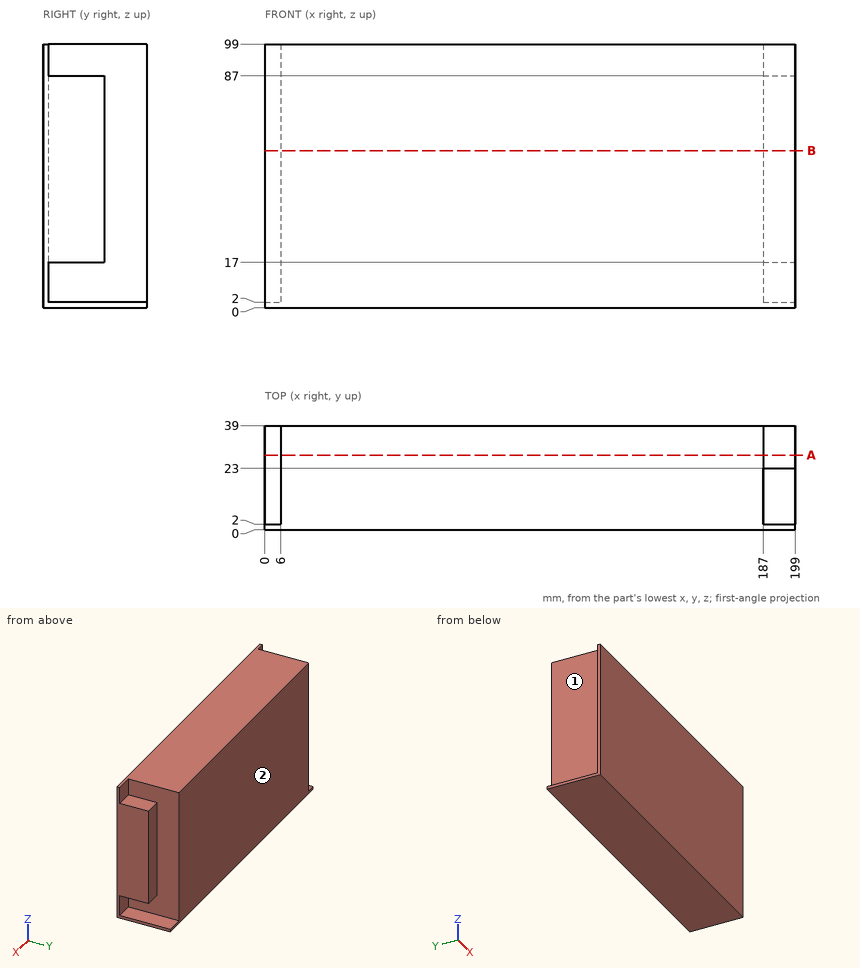
Study the drawing (mm; zero at the part's minimum x, y, z) and answer. A direction names the side the tool comes from. Round coordinates to 2 decimals unless told otherwise and drop trailing zeros. Write each loop counter-clockwise with the first axis right and the second up, starting at its lowest first coordinate (ties: lowest second). Pieces come first, ordered by that corner, then holes.
1) A cutting plane is placed at A-A on y = 28. Determine the outline of the cut face in (x, z).
2) Flat-ended cylindrical pins translate along their axes: P1, Ø13, axis at x = 195, y = 17, coming from the -Z side; P2, Ø3, axis at y = 11.5, z = 51, coming from the -X side; P3, Ø9.5, axis at x = 195.5, z = 96, coming from the +Y side; P4, Ø3.5, axis at x = 190.5, y = 14, coming from the +Z side. Find the tip coordinate at first contact, or state that the pin passes through.
3) Consider probe 1 along X at (y, z) = (17, 17.5); probe 2 along X at (y, z) = (7.5, 8.5). Determine where each line is inside the solid, lowest interval first.
4) A cutting plane is placed at B-B on z = 59. Determine the outline of the cut face in (x, y).
5) Which of the six approach directions +Z, -Z, +X, -X, +Y, -Y give full straight-line access (tool end or side, diameter ignored) to the marked faces 1 and 2?
Entries:
1. outline: (0, 0) - (199, 0) - (199, 2) - (187, 2) - (187, 99) - (6, 99) - (6, 2) - (0, 2) - close
2. P1: stops at z = 0
2. P2: stops at x = 6
2. P3: stops at y = 2
2. P4: stops at z = 87
3. probe 1: x = 6 to 199
3. probe 2: x = 6 to 187
4. outline: (0, 0) - (199, 0) - (199, 23) - (187, 23) - (187, 39) - (6, 39) - (6, 2) - (0, 2) - close
5. face 1: +Z, -X, +Y
5. face 2: +Z, -Z, +X, -X, +Y
